```python
from build123d import *

# Parameters (mm, degrees)
F0_W      = 62
F0_H      = 40.32
F1_DEPTH  = 11.25
F2_W      = 25
F2_H      = 9.1
F3_DEPTH  = 3.2
F4_W      = 10.9982
F4_H      = 3.1144623497
F4_H_2    = 3.5855376503
F5_DEPTH  = 1.25
F6_R      = 3.81
F7_R      = 2
F8_DEPTH  = 15.24
F10_DEPTH = 4.25


with BuildPart() as f1:
    # F0 (on Front) → F1 (new body)
    with BuildSketch(Plane.XZ):
        Rectangle(F0_W, F0_H)
    extrude(amount=F1_DEPTH)

    # F2 (on face) → F3 (cut)
    with BuildSketch(Plane.XZ.offset(11.25)):
        Rectangle(F2_W, F2_H)
    extrude(amount=-F3_DEPTH, mode=Mode.SUBTRACT)

    # F4 (on face) → F5 (join)
    with BuildSketch(Plane.XZ.offset(11.25)):
        with Locations((-7.0009, 2.9927688252)):
            Rectangle(F4_W, F4_H)
        with Locations((-7.0009, -2.7572311748)):
            Rectangle(F4_W, F4_H_2)
    extrude(amount=-F5_DEPTH)

    # F6
    f6_edges = [f1.edges().sort_by_distance(p)[0] for p in [
        (-31, -5.625, 20.16),
        (31, -5.625, 20.16),
        (31, -5.625, -20.16),
        (-31, -5.625, -20.16),
    ]]
    fillet(f6_edges, radius=F6_R)

    # F7 (on face) → F8 (cut)
    with BuildSketch(Plane.XZ.offset(11.25)):
        with Locations((-24.2824, 0.5)):
            Circle(F7_R)
        with Locations((24.2824, 0.5)):
            Circle(F7_R)
    extrude(amount=-F8_DEPTH, mode=Mode.SUBTRACT)

    # F9 (on face) → F10 (cut)
    with BuildSketch(Plane.XZ.offset(11.25)):
        Polygon((-24.3669678343, -4.8146678066), (-20.021959685, -2.3119505341), (-20.0168723469, 2.7022955391), (-24.356793158, 5.2138243397), (-28.7018013073, 2.7111070672), (-28.7068886454, -2.3031390059), align=None)
        Polygon((24.3045226557, -4.7588889519), (28.6495308049, -2.2561716794), (28.654618143, 2.7580743938), (24.3146973319, 5.2696031944), (19.9696891827, 2.7668859219), (19.9646018445, -2.2473601513), align=None)
    extrude(amount=-F10_DEPTH, mode=Mode.SUBTRACT)


solid = f1.part
```
Source: CAD feature listing. Evaluate the final solid. Frame: model axes, mm. A direction names the side the tool comes from. Give positions to 0.01 mm unless a question says otherwise; leave off trailing zeros. Order: outer loops, then holes, each group sorted by start corner. A loop starts at its lowest first (then second) coordinate and runs counter-clockwise, first axis right, second up.
(1) Access query for faces 1 (the face through (29.854, -5.704, -19.074)), 2 (the face through (-12.5, -9, 0)), 3 (the face through (-1.502, -11, -3)). Directions: +Z, -Z, +X, -X, +Y, -Y. A direction counts if a zero-diameter tool reaches every point of the face in a straight line with its end or side. Return the directions, or none.
(2) Pull-direction query (Y, two-part tool) for faces 4 (the face through (0, -11.25, 5)), 5 (the face through (-22.156, -9.155, 3.94)), 6 (the face through (-7, -10, 3)); classes: +Y half, -Y half, draft (parallel to the pull), parting line (faces both ways), or undercut.
(3) Contact query for flat-ended pins moving along their axis: P1, Ø7, axis at x = 24, z = 0, coming from the -Y side; P2, Ø3.5, axis at x = 24.28, z = 0.5, coming from the -Y side. Output: stop coordinate, or through.
(4) Section query B-B (z = 0.5). Return the cut outline in (x, y), plus the area to 3 significant figures.
(5) Section query C-C (x = 11). Return the cut outline in (y, z), plus the area to 3 significant figures.
(6) Material intervals for line 1 along X through (y, z) = (-7.25, -1.5); line 2 along Z through (x, y) = (8.5, -8.75); line 3 along X through (y, z) = (-9.25, -2), sorted ascending.
(7) Section query A-A (y = -1). Return the cut outline in (x, z), plus the area to 3 significant figures.
(8) Section query D-D (x = -25). Return the cut outline in (y, z).
Outcome:
1. face 1: -Z, +X, +Y, -Y
1. face 2: none
1. face 3: -Y
2. face 4: -Y half
2. face 5: draft
2. face 6: undercut
3. P1: stops at y = -7
3. P2: passes through
4. outline: (-31, -11.25) - (-28.7, -11.25) - (-28.7, -7) - (-26.28, -7) - (-26.28, 0) - (-31, 0) - close; (-22.28, -7) - (-20.02, -7) - (-20.02, -11.25) - (-12.5, -11.25) - (-12.5, -8.05) - (12.5, -8.05) - (12.5, -11.25) - (19.97, -11.25) - (19.97, -7) - (22.28, -7) - (22.28, 0) - (-22.28, 0) - close; (26.28, -7) - (28.65, -7) - (28.65, -11.25) - (31, -11.25) - (31, 0) - (26.28, 0) - close
4. area: 488 mm2
5. outline: (-11.25, -20.16) - (0, -20.16) - (0, 20.16) - (-11.25, 20.16) - (-11.25, 4.55) - (-8.05, 4.55) - (-8.05, -4.55) - (-11.25, -4.55) - close
5. area: 424 mm2
6. line 1: x = -31 to -28.71, -20.02 to 19.97, 28.65 to 31
6. line 2: z = -20.16 to -4.55, 4.55 to 20.16
6. line 3: x = -31 to -28.71, -20.02 to -12.5, 12.5 to 19.96, 28.65 to 31
7. outline: (-31, -16.35) arc R3.81 ccw to (-27.19, -20.16) - (27.19, -20.16) arc R3.81 ccw to (31, -16.35) - (31, 16.35) arc R3.81 ccw to (27.19, 20.16) - (-27.19, 20.16) arc R3.81 ccw to (-31, 16.35) - close; hole circle Ø4 at (-24.28, 0.5); hole circle Ø4 at (24.28, 0.5)
7. area: 2,460 mm2
8. outline: (-11.25, -20.16) - (0, -20.16) - (0, -1.37) - (-7, -1.37) - (-7, -4.45) - (-11.25, -4.45) - close; (-11.25, 4.84) - (-7, 4.84) - (-7, 2.37) - (0, 2.37) - (0, 20.16) - (-11.25, 20.16) - close
